Source: CAD feature listing. Evaluate the final solid. Frame: model axes, mm. Round coordinates to 2 decimals unless told otherwise and drop trailing zeros. Order: outer loops, then holes, each group sorted by start corner. A loop starts at its lowest first (then second) coordinate and runs counter-clockwise, first axis right, second up. Notation, with made-up numbers: (-39.75, 24) - (-26.75, 24) arc R23 cw to (-26.75, 38) - close; hole circle Ø5 at (2, 37). An arc over 180 degrees is marked (long way). Use one line per item in the form item = value. Start each with the question number.
Q1. Ray query, line 1 (Y direction, x = 14, z = 1.4); line 2 (Y direction, x = 20, z = 0.6); line 3 (X direction, y = -6, z = 1.8). Return the intervals inside material, ascending. Write a range as [from, to].
Q2. Cut plane A-A, the plane y = 0. Return the cut outline in (x, z).
Q3. Pin query (flat end, axial travel): pin 1 Ø6 at (x, y) = (20, 0) entering from +Z. Return the tip coordinate at first contact, or that it passes through.
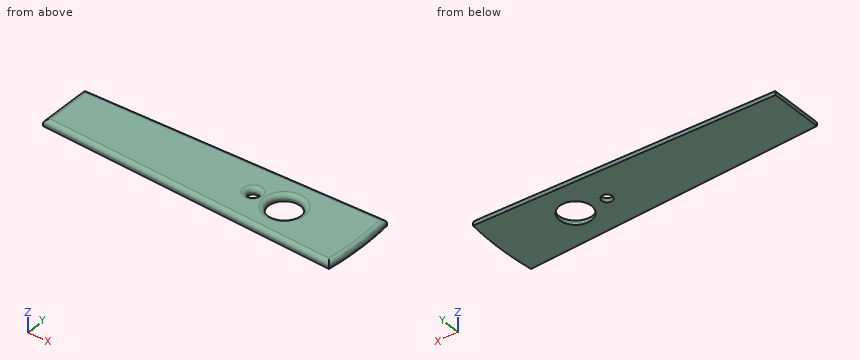
from build123d import *

# Parameters (mm, degrees)
F0_R     = 2.5
F0_R_2   = 7.5
F1_DEPTH = 3
F2_R     = 2


with BuildPart() as f1:
    # F0 (on Top) → F1 (new body)
    with BuildSketch(Plane.XY):
        with BuildLine():
            Line((70, 17.5), (-70, 12.5))
            Line((-70, 12.5), (-70, -12.5))
            Line((-70, -12.5), (70, -17.5))
            ThreePointArc((70, -17.5), (71.089511, 0), (70, 17.5))
        make_face()
        with Locations((20, 0)):
            Circle(F0_R, mode=Mode.SUBTRACT)
        with Locations((35, 0)):
            Circle(F0_R_2, mode=Mode.SUBTRACT)
    extrude(amount=F1_DEPTH)

    # F2
    f2_edges = [f1.edges().sort_by_distance(p)[0] for p in [
        (0, 15, 3),
        (-70, 0, 3),
        (0, -15, 3),
        (71.089511, 0, 3),
        (17.5, 0, 3),
        (27.5, 0, 3),
    ]]
    fillet(f2_edges, radius=F2_R)


solid = f1.part
Completed:
q1.line_1 = [-15.46, 15.46]
q1.line_2 = [-15.71, -2.5], [2.5, 15.71]
q1.line_3 = [-69.83, 30.23], [39.77, 70.79]
q2.outline = (-70, 0) - (17.5, 0) - (17.5, 1) arc R2 ccw to (15.5, 3) - (-68, 3) arc R2 ccw to (-70, 1) - close; (22.5, 0) - (27.5, 0) - (27.5, 1) arc R2 ccw to (25.5, 3) - (24.5, 3) arc R2 ccw to (22.5, 1) - close; (42.5, 0) - (71.09, 0) - (71.09, 1) arc R2 ccw to (69.09, 3) - (44.5, 3) arc R2 ccw to (42.5, 1) - close
q3.pin_1 = 2.32
